Part model, mm, in its own coordinate system. A direction names the side the tool comes from. Round coordinates to 2 decimals unless told otherwise and drop trailing zeros. Order: outer loops, then holes, each group sorted by start corner. A loop starts at its lowest first (then second) coordinate and runs counter-clockwise, first axis right, second up. Notation, with made-up numbers: M 48,79.5 L 60,79.5 A36 ccw 60,116.5 Z; hole C 2,31 d2. An arc over 180 degrees is marked long. Write each question's results on one line, items separated by ' | '. Start each with the question number.
1. Probe L1, parallel to Y at x = -9.75, z = 2.05; L2, parallel to X at y = -8.5, z = 7.25; L3, parallel to Y at x = 0, z = 1.1. List the from-to ranges inside material, lowest first. Write a range as [from, to].
2. Drop flat-ended pins along their axis: pin 1 Ø0.8 at (y, z) = (6.5, 1) entering from -X; pin 2 Ø9 at (x, y) = (-39, 0) entering from -Z; pin 3 Ø3 at (y, z) = (-21.5, 4.5) entering from +X. Give the stop position or say it passes through.
3. Which spindle directions (+Z, -Z, +X, -X, +Y, -Y) get a long thin tool onto all of the face, cutting with end or side? Do faces 1 (the face through (-11.34, -19.72, 5.74)), 2 (the face through (-31.75, 7, 1)), 3 (the face through (-8.25, 6, 7)), 4 (the face through (-19, -8, 0)), 5 (the face through (-25, -11, 6.5)). Say none if no direction does.
4. Two-plate mould, pull along Y, no slides. Class faces 6 (the face through (1.64, -12.16, 1.48)), 7 (the face through (-20, -25.887, 4)), 8 (the face through (7.859, 4.385, 3.944)): +Y half, -Y half, draft (parallel to the pull), parting line (faces both ways), or undercut.
5. Band-saw the part on C-C, the plane y = 0. List the corners of the cut face in (x, z).
6. Band-saw the part on D-D, the plane x = -4.5. List the corners of the cut face in (y, z).
7. Band-saw the part on A-A, the plane z = 2. Give the number of separate pieces and of enclosed holes in the cut face, then the cut area to 3 significant figures.
```python
from build123d import *

# Parameters (mm, degrees)
SKETCH1_R           = 7.5
BOSS_EXTRUDE1_DEPTH = 5
SKETCH2_R           = 7.5
BOSS_EXTRUDE2_DEPTH = 1.5
BOSS_EXTRUDE3_DEPTH = 1.5
SKETCH9_W           = 3
SKETCH9_H           = 6
CUT_EXTRUDE4_DEPTH  = 3
SKETCH4_W           = 5
SKETCH4_H           = 1.5
CUT_EXTRUDE5_DEPTH  = 3


with BuildPart() as part:
    # Sketch1 → Boss-Extrude1 (new body)
    with BuildSketch(Plane.XY):
        with BuildLine():
            Line((7.794228634, -4.5), (-1.955771366, -21.387495374))
            ThreePointArc((-1.955771366, -21.387495374), (-5.25, -24.681724008), (-9.75, -25.887495374))
            Line((-9.75, -25.887495374), (-29.25, -25.887495374))
            ThreePointArc((-29.25, -25.887495374), (-33.75, -24.681724008), (-37.044228634, -21.387495374))
            Line((-37.044228634, -21.387495374), (-46.794228634, -4.5))
            ThreePointArc((-46.794228634, -4.5), (-46.794228634, 4.5), (-39, 9))
            Line((-39, 9), (0, 9))
            ThreePointArc((0, 9), (7.794228634, 4.5), (7.794228634, -4.5))
        make_face()
        with Locations((-29.25, -16.887495374)):
            Circle(SKETCH1_R, mode=Mode.SUBTRACT)
        with Locations((-19.5, 0)):
            Circle(SKETCH1_R, mode=Mode.SUBTRACT)
        Circle(SKETCH1_R, mode=Mode.SUBTRACT)
        with Locations((-9.75, -16.887495374)):
            Circle(SKETCH1_R, mode=Mode.SUBTRACT)
        with Locations((-39, 0)):
            Circle(SKETCH1_R, mode=Mode.SUBTRACT)
    extrude(amount=BOSS_EXTRUDE1_DEPTH)

    # Sketch2 → Boss-Extrude2 (add)
    # profile 1 of 6: a face of its own
    with BuildSketch(Plane.XY.offset(5)):
        with BuildLine():
            Line((-1.955771366, -21.387495374), (7.794228634, -4.5))
            ThreePointArc((7.794228634, -4.5), (7.794228634, 4.5), (0, 9))
            Line((0, 9), (-39, 9))
            ThreePointArc((-39, 9), (-46.794228634, 4.5), (-46.794228634, -4.5))
            Line((-46.794228634, -4.5), (-37.044228634, -21.387495374))
            ThreePointArc((-37.044228634, -21.387495374), (-33.75, -24.681724008), (-29.25, -25.887495374))
            Line((-29.25, -25.887495374), (-9.75, -25.887495374))
            ThreePointArc((-9.75, -25.887495374), (-5.25, -24.681724008), (-1.955771366, -21.387495374))
        make_face()
        Circle(SKETCH2_R, mode=Mode.SUBTRACT)
        with Locations((-19.5, 0)):
            Circle(SKETCH2_R, mode=Mode.SUBTRACT)
        with Locations((-39, 0)):
            Circle(SKETCH2_R, mode=Mode.SUBTRACT)
        with Locations((-29.25, -16.887495374)):
            Circle(SKETCH2_R, mode=Mode.SUBTRACT)
        with Locations((-9.75, -16.887495374)):
            Circle(SKETCH2_R, mode=Mode.SUBTRACT)
    # profile 2 of 6: a face of its own
    with BuildSketch(Plane.XY.offset(5)):
        with Locations((-9.75, -16.887495374)):
            Circle(SKETCH2_R)
        with BuildLine():
            ThreePointArc((-13.540063509, -18.452077936), (-14.223076211, -18.635090638), (-14.040063509, -19.31810334))
            Line((-14.040063509, -19.31810334), (-9.709936491, -21.81810334))
            ThreePointArc((-9.709936491, -21.81810334), (-9.026923789, -21.635090638), (-9.209936491, -20.952077936))
            Line((-9.209936491, -20.952077936), (-13.540063509, -18.452077936))
        make_face(mode=Mode.SUBTRACT)
    # profile 3 of 6: a face of its own
    with BuildSketch(Plane.XY.offset(5)):
        Circle(SKETCH2_R)
        with BuildLine():
            ThreePointArc((-0.040063509, 4.930607966), (-0.723076211, 4.747595264), (-0.540063509, 4.064582562))
            Line((-0.540063509, 4.064582562), (3.790063509, 1.564582562))
            ThreePointArc((3.790063509, 1.564582562), (4.473076211, 1.747595264), (4.290063509, 2.430607966))
            Line((4.290063509, 2.430607966), (-0.040063509, 4.930607966))
        make_face(mode=Mode.SUBTRACT)
    # profile 4 of 6: a face of its own
    with BuildSketch(Plane.XY.offset(5)):
        with Locations((-19.5, 0)):
            Circle(SKETCH2_R)
        with BuildLine():
            ThreePointArc((-19.540063509, 4.930607966), (-20.223076211, 4.747595264), (-20.040063509, 4.064582562))
            Line((-20.040063509, 4.064582562), (-15.709936491, 1.564582562))
            ThreePointArc((-15.709936491, 1.564582562), (-15.026923789, 1.747595264), (-15.209936491, 2.430607966))
            Line((-15.209936491, 2.430607966), (-19.540063509, 4.930607966))
        make_face(mode=Mode.SUBTRACT)
    # profile 5 of 6: a face of its own
    with BuildSketch(Plane.XY.offset(5)):
        with Locations((-29.25, -16.887495374)):
            Circle(SKETCH2_R)
        with BuildLine():
            ThreePointArc((-33.040063509, -18.452077936), (-33.723076211, -18.635090638), (-33.540063509, -19.31810334))
            Line((-33.540063509, -19.31810334), (-29.209936491, -21.81810334))
            ThreePointArc((-29.209936491, -21.81810334), (-28.526923789, -21.635090638), (-28.709936491, -20.952077936))
            Line((-28.709936491, -20.952077936), (-33.040063509, -18.452077936))
        make_face(mode=Mode.SUBTRACT)
    # profile 6 of 6: a face of its own
    with BuildSketch(Plane.XY.offset(5)):
        with Locations((-39, 0)):
            Circle(SKETCH2_R)
        with BuildLine():
            ThreePointArc((-42.790063509, -1.564582562), (-43.473076211, -1.747595264), (-43.290063509, -2.430607966))
            Line((-43.290063509, -2.430607966), (-38.959936491, -4.930607966))
            ThreePointArc((-38.959936491, -4.930607966), (-38.276923789, -4.747595264), (-38.459936491, -4.064582562))
            Line((-38.459936491, -4.064582562), (-42.790063509, -1.564582562))
        make_face(mode=Mode.SUBTRACT)
        with BuildLine():
            ThreePointArc((-39.040063509, 4.930607966), (-39.723076211, 4.747595264), (-39.540063509, 4.064582562))
            Line((-39.540063509, 4.064582562), (-35.209936491, 1.564582562))
            ThreePointArc((-35.209936491, 1.564582562), (-34.526923789, 1.747595264), (-34.709936491, 2.430607966))
            Line((-34.709936491, 2.430607966), (-39.040063509, 4.930607966))
        make_face(mode=Mode.SUBTRACT)
    extrude(amount=BOSS_EXTRUDE2_DEPTH)

    # Sketch3 → Boss-Extrude3 (add)
    with BuildSketch(Plane.XY.offset(6.5)):
        with BuildLine():
            ThreePointArc((-39, 9), (-46.794228634, 4.5), (-46.794228634, -4.5))
            Line((-46.794228634, -4.5), (-46.144709581, -5.625))
            Line((-46.144709581, -5.625), (-38.985335738, 6.775399247))
            Line((-38.985335738, 6.775399247), (-33.139664262, 3.400399247))
            Line((-33.139664262, 3.400399247), (-42.247595264, -12.375))
            Line((-42.247595264, -12.375), (-37.044228634, -21.387495374))
            ThreePointArc((-37.044228634, -21.387495374), (-36.712405778, -21.918648323), (-36.344447387, -22.425438699))
            Line((-36.344447387, -22.425438699), (-34.985335738, -20.07138827))
            Line((-34.985335738, -20.07138827), (-19.610335738, 6.558892896))
            Line((-19.610335738, 6.558892896), (-13.764664262, 3.183892896))
            Line((-13.764664262, 3.183892896), (-29.139664262, -23.44638827))
            Line((-29.139664262, -23.44638827), (-30.498775911, -25.800438699))
            ThreePointArc((-30.498775911, -25.800438699), (-29.875903375, -25.865704826), (-29.25, -25.887495374))
            Line((-29.25, -25.887495374), (-18.84326674, -25.887495374))
            Line((-18.84326674, -25.887495374), (-15.485335738, -20.07138827))
            Line((-15.485335738, -20.07138827), (-0.110335738, 6.558892896))
            Line((-0.110335738, 6.558892896), (5.735335738, 3.183892896))
            Line((5.735335738, 3.183892896), (-9.639664262, -23.44638827))
            Line((-9.639664262, -23.44638827), (-11.049038106, -25.887495374))
            Line((-11.049038106, -25.887495374), (-9.75, -25.887495374))
            ThreePointArc((-9.75, -25.887495374), (-5.25, -24.681724008), (-1.955771366, -21.387495374))
            Line((-1.955771366, -21.387495374), (7.794228634, -4.5))
            ThreePointArc((7.794228634, -4.5), (7.794228634, 4.5), (0, 9))
            Line((0, 9), (-39, 9))
        make_face()
    extrude(amount=BOSS_EXTRUDE3_DEPTH)

    # Sketch9 → Cut-Extrude4 (cut)
    with BuildSketch(Plane.XY.offset(8)):
        with Locations((-29.25, 6)):
            Rectangle(SKETCH9_W, SKETCH9_H)
        with Locations((-9.75, 6)):
            Rectangle(SKETCH9_W, SKETCH9_H)
    extrude(amount=-CUT_EXTRUDE4_DEPTH, mode=Mode.SUBTRACT)

    # Sketch4 → Cut-Extrude5 (cut)
    with BuildSketch(Plane(origin=(0, 0, 0), x_dir=(-1, 0, 0), z_dir=(0, 0, -1))):
        Polygon((-2.870190528, -10.028684177), (-0.370190528, -14.358811196), (0.928847577, -13.608811196), (-1.571152423, -9.278684177), align=None)
        with Locations((9.75, 6.75)):
            Rectangle(SKETCH4_W, SKETCH4_H)
        with Locations((29.25, 6.75)):
            Rectangle(SKETCH4_W, SKETCH4_H)
        Polygon((39.370190528, -14.358811196), (41.870190528, -10.028684177), (40.571152423, -9.278684177), (38.071152423, -13.608811196), align=None)
        with Locations((19.5, -23.637495374)):
            Rectangle(SKETCH4_W, SKETCH4_H)
    extrude(amount=-CUT_EXTRUDE5_DEPTH, mode=Mode.SUBTRACT)


solid = part.part
```
Solution:
1) L1: [-25.89, -24.39], [-9.39, 6], [7.5, 9] | L2: [-40.01, -28.3], [-20.51, -8.8], [-1.01, 5.48] | L3: [-18, -14.15], [-12, -7.5], [7.5, 9]
2) pin 1: x = -45.62 | pin 2: z = 5 | pin 3: x = -1.15
3) face 1: +Z, -Z | face 2: -Z | face 3: +Z, +Y | face 4: -Z, +X, -X, +Y, -Y | face 5: +Z
4) face 6: undercut | face 7: -Y half | face 8: parting line
5) outline: M -48,0 L -46.5,0 L -46.5,5 L -31.5,5 L -31.5,0 L -27,0 L -27,5 L -12,5 L -12,0 L -7.5,0 L -7.5,5 L 7.5,5 L 7.5,0 L 9,0 L 9,8 L 3.9,8 L 3.9,6.5 L -3.9,6.5 L -3.9,8 L -15.6,8 L -15.6,6.5 L -23.4,6.5 L -23.4,8 L -35.1,8 L -35.1,6.5 L -42.9,6.5 L -42.9,8 L -48,8 Z
6) outline: M -24.2,0 L -22.24,0 L -22.24,5 L -11.53,5 L -11.53,0 L -6,0 L -6,5 L 6,5 L 6,0 L 9,0 L 9,8 L -1.04,8 L -1.04,6.5 L -14.54,6.5 L -14.54,8 L -24.2,8 Z
7) separate pieces: 1 | enclosed holes: 10 | area: 705 mm^2
